from build123d import *

# Parameters (mm, degrees)
SALIENTE_EXTRUIR1_DEPTH = 0.1


with BuildPart() as part:
    # Model → Saliente-Extruir1 (new body)
    with BuildSketch(Plane.XY):
        with BuildLine():
            Line((24.573492595, 10.397787824), (16.586059329, 8.480394017))
            Line((16.586059329, 8.480394017), (15.223673977, 21.22645362))
            ThreePointArc((15.223673977, 21.22645362), (9.038896644, 20.100865764), (2.933605753, 18.6029199))
            Line((2.933605753, 18.6029199), (19.512585392, 31.480394017))
            Line((19.512585392, 31.480394017), (24.573492595, 10.397787824))
        make_face()
    extrude(amount=SALIENTE_EXTRUIR1_DEPTH)


solid = part.part
CAD build for the part. Positions are in the model's coordinates, mm. Coordinates: 2 decimals unless noted, no trailing zeros. Write each loop counter-clockwise with the first axis right and the second up, starting at its lowest first coordinate (ties: lowest second). Pieces come first, ordered by that corner, then holes. Notation, with made-up numbers: M 20.25,-40 L 74.25,-40 A13 ccw 74.25,-29 Z; hole C 40.25,68 d5. An arc over 180 degrees is marked long. Answer as a JSON object with one key per item and string values. Group by question number.
1) Saw through at C-C (x = 7.75). Write the cut outline in (y, z).
2) Saw through at A-A (y = 20). Write the cut outline in (x, z).
3) Saw through at D-D (y = 17.5). Write the cut outline in (x, z), plus the area to 3 significant figures.
4) Wall check: line 1 (Y direction, x = 11.25, z = 0.05); line 2 (X direction, y = 14.25, z = 0.05); line 3 (Y direction, x = 17, z = 0.05). Give the ranges that are in metal, low to high. Write a range as from..to.
5) Saw through at B-B (z = 0.05). Write the cut outline in (x, y), plus the area to 3 significant figures.
Values follow:
{
 "1": {"outline": "M 19.82,0 L 22.34,0 L 22.34,0.1 L 19.82,0.1 Z"},
 "2": {"outline": "M 4.73,0 L 8.57,0 L 8.57,0.1 L 4.73,0.1 Z; M 15.35,0 L 22.27,0 L 22.27,0.1 L 15.35,0.1 Z"},
 "3": {"outline": "M 15.62,0 L 22.87,0 L 22.87,0.1 L 15.62,0.1 Z", "area": "0.725 mm2"},
 "4": {"line 1": "y = 20.55..25.06", "line 2": "x = 15.97..23.65", "line 3": "y = 8.58..29.53"},
 "5": {"outline": "M 2.93,18.6 A103.79 cw 15.22,21.23 L 16.59,8.48 L 24.57,10.4 L 19.51,31.48 Z", "area": "179 mm2"}
}
